Source: CAD feature listing. Evaluate the final solid. Frame: model axes, mm. A direction names the side the tool comes from. Coordinates: 2 decimals unless noted, no trailing zeros. Write each loop counter-clockwise with the first axis right and the second up, starting at its lowest first coordinate (ties: lowest second). Pieces come first, ordered by that corner, then holes. Notation, with made-up numbers: M -20,25 L 16,25 A13 cw 16,45 Z; hole C 39,-21 d9. An arc over 180 degrees is marked long. Write item = value, one per line. Start each with the question number.
1. Section query A-A (x = -20). Give the number of separate pieces and of enclosed holes in the cut face, then the cut area to 4 significant figures.
2. Section query C-C (z = 35). Output: boundary loops of the cut face in (x, y).
3. Access query for faces 4 (the face through (-5, 30, 53)), 5 (the face through (-33, 15, 37)), 6 (the face through (-8, 30, 42)), 7 (the face through (-20, 16, 47)), 8 (the face through (-33.5, 6, 51)). Directions: +Z, -Z, +X, -X, +Y, -Y. A direction counts if a zero-diameter tool reaches every point of the face in a straight line with its end or side. Return the directions, or none.
4. Pin query (flat end, axial travel): pin 1 Ø3.5 at (x, y) = (-8, 29.5) entering from +Z; pin 2 Ø2.5 at (x, y) = (-30, 7.5) entering from +Z; pin 3 Ø4 at (x, z) = (-16, 21.5) entering from +Y. Return the tip coordinate at first contact, or that it passes through.
5. Line query: line 1 along Z through (x, y) = (-9, 20); line 2 along Z through (x, y) = (-11.5, 31); line 3 along X through (y, z) = (3.5, 44.5). Output: solid intervals per line, ascending.
6. Pull-direction query (X, two-part tool) for faces 1 (the face through (0, 20, 28)), 2 (the face through (-30, 17, 31)), 3 (the face through (-9.748, 30.099, 55.028)); classes: pulls with the +X half, pulls with the -X half, needs draft (parallel to the pull), parting line crosses it, or undercut.
```python
from build123d import *

# Parameters (mm, degrees)
ESQUISSE1_W              = 40
ESQUISSE1_H              = 40
BOSS_EXTRU_1_DEPTH       = 50
ESQUISSE2_R              = 5
ENL_V_MAT_EXTRU_1_DEPTH  = 41
ESQUISSE3_R              = 5
ENL_V_MAT_EXTRU_2_DEPTH  = 41
ESQUISSE4_W              = 22
ESQUISSE4_H              = 14
ENL_V_MAT_EXTRU_3_DEPTH  = 29
ESQUISSE5_W              = 14
ESQUISSE5_H              = 20
ENL_V_MAT_EXTRU_4_DEPTH  = 29
ESQUISSE6_W              = 20
ESQUISSE6_H              = 14
ENL_V_MAT_EXTRU_5_DEPTH  = 24
ESQUISSE7_W              = 14
ESQUISSE7_H              = 22
ENL_V_MAT_EXTRU_6_DEPTH  = 24
ESQUISSE10_R             = 11
ENL_V_MAT_EXTRU_9_DEPTH  = 7
ESQUISSE11_R             = 12.5
ENL_V_MAT_EXTRU_10_DEPTH = 1.5
ESQUISSE14_R             = 11
ENL_V_MAT_EXTRU_11_DEPTH = 7
ESQUISSE15_R             = 12.5
ENL_V_MAT_EXTRU_12_DEPTH = 1.5
ESQUISSE16_W             = 40
ESQUISSE16_H             = 40
BOSS_EXTRU_2_DEPTH       = 7
ESQUISSE17_R             = 2.25
ENL_V_MAT_EXTRU_13_DEPTH = 15
ESQUISSE18_W             = 7
ESQUISSE18_H             = 3
ENL_V_MAT_EXTRU_14_DEPTH = 12
ESQUISSE19_W             = 3.5
ESQUISSE19_H             = 7.5
ENL_V_MAT_EXTRU_15_DEPTH = 12


with BuildPart() as part:
    # Esquisse1 → Boss.-Extru.1 (new body)
    with BuildSketch(Plane.XY):
        with Locations((-20, 20)):
            Rectangle(ESQUISSE1_W, ESQUISSE1_H)
    extrude(amount=BOSS_EXTRU_1_DEPTH)

    # Esquisse2 → Enlèv. mat.-Extru.1 (cut, through all)
    with BuildSketch(Plane(origin=(0, 40, 0), x_dir=(1, 0, 0), z_dir=(0, 1, 0))):
        with Locations(Location((-20, -15, 0), (0, 0, 270))):  # turned: the seam where the file's is
            Circle(ESQUISSE2_R)
    extrude(amount=-ENL_V_MAT_EXTRU_1_DEPTH, mode=Mode.SUBTRACT)

    # Esquisse3 → Enlèv. mat.-Extru.2 (cut, through all)
    with BuildSketch(Plane.ZY.offset(40)):
        with Locations((35, 20)):
            Circle(ESQUISSE3_R)
    extrude(amount=-ENL_V_MAT_EXTRU_2_DEPTH, mode=Mode.SUBTRACT)

    # Esquisse4 → Enlèv. mat.-Extru.3 (cut)
    with BuildSketch(Plane.ZY.offset(40)):
        with Locations((11, 20)):
            Rectangle(ESQUISSE4_W, ESQUISSE4_H)
    extrude(amount=-ENL_V_MAT_EXTRU_3_DEPTH, mode=Mode.SUBTRACT)

    # Esquisse5 → Enlèv. mat.-Extru.4 (cut)
    with BuildSketch(Plane.XZ):
        with Locations((-20, 35)):
            Rectangle(ESQUISSE5_W, ESQUISSE5_H)
    extrude(amount=-ENL_V_MAT_EXTRU_4_DEPTH, mode=Mode.SUBTRACT)

    # Esquisse6 → Enlèv. mat.-Extru.5 (cut)
    with BuildSketch(Plane(origin=(0, 0, 0), x_dir=(0, 0, -1), z_dir=(1, 0, 0))):
        with Locations((-15, 20)):
            Rectangle(ESQUISSE6_W, ESQUISSE6_H)
    extrude(amount=-ENL_V_MAT_EXTRU_5_DEPTH, mode=Mode.SUBTRACT)

    # Esquisse7 → Enlèv. mat.-Extru.6 (cut)
    with BuildSketch(Plane(origin=(0, 40, 0), x_dir=(1, 0, 0), z_dir=(0, 1, 0))):
        with Locations((-20, -39)):
            Rectangle(ESQUISSE7_W, ESQUISSE7_H)
    extrude(amount=-ENL_V_MAT_EXTRU_6_DEPTH, mode=Mode.SUBTRACT)

    # Esquisse10 → Enlèv. mat.-Extru.9 (cut)
    with BuildSketch(Plane(origin=(0, 40, 0), x_dir=(1, 0, 0), z_dir=(0, 1, 0))):
        with Locations(Location((-20, -15, 0), (0, 0, 270))):  # turned: the seam where the file's is
            Circle(ESQUISSE10_R)
    extrude(amount=-ENL_V_MAT_EXTRU_9_DEPTH, mode=Mode.SUBTRACT)

    # Esquisse11 → Enlèv. mat.-Extru.10 (cut)
    with BuildSketch(Plane(origin=(0, 40, 0), x_dir=(1, 0, 0), z_dir=(0, 1, 0))):
        with Locations(Location((-20, -15, 0), (0, 0, 270))):  # turned: the seam where the file's is
            Circle(ESQUISSE11_R)
    extrude(amount=-ENL_V_MAT_EXTRU_10_DEPTH, mode=Mode.SUBTRACT)

    # Esquisse14 → Enlèv. mat.-Extru.11 (cut)
    with BuildSketch(Plane.ZY.offset(40)):
        with Locations((35, 20)):
            Circle(ESQUISSE14_R)
    extrude(amount=-ENL_V_MAT_EXTRU_11_DEPTH, mode=Mode.SUBTRACT)

    # Esquisse15 → Enlèv. mat.-Extru.12 (cut)
    with BuildSketch(Plane.ZY.offset(40)):
        with Locations((35, 20)):
            Circle(ESQUISSE15_R)
    extrude(amount=-ENL_V_MAT_EXTRU_12_DEPTH, mode=Mode.SUBTRACT)

    # Esquisse16 → Boss.-Extru.2 (add)
    with BuildSketch(Plane.XY.offset(50)):
        with Locations((-20, 20)):
            Rectangle(ESQUISSE16_W, ESQUISSE16_H)
    extrude(amount=BOSS_EXTRU_2_DEPTH)

    # Esquisse17 → Enlèv. mat.-Extru.13 (cut)
    with BuildSketch(Plane.XY.offset(57)):
        with Locations((-30, 7.5)):
            Circle(ESQUISSE17_R)
        with Locations((-7.5, 30)):
            Circle(ESQUISSE17_R)
    extrude(amount=-ENL_V_MAT_EXTRU_13_DEPTH, mode=Mode.SUBTRACT)

    # Esquisse18 → Enlèv. mat.-Extru.14 (cut)
    with BuildSketch(Plane.XZ):
        with Locations((-30, 51.5)):
            Rectangle(ESQUISSE18_W, ESQUISSE18_H)
    extrude(amount=-ENL_V_MAT_EXTRU_14_DEPTH, mode=Mode.SUBTRACT)

    # Esquisse19 → Enlèv. mat.-Extru.15 (cut)
    with BuildSketch(Plane(origin=(0, 0, 0), x_dir=(0, 0, -1), z_dir=(1, 0, 0))):
        with Locations((-51.25, 30)):
            Rectangle(ESQUISSE19_W, ESQUISSE19_H)
    extrude(amount=-ENL_V_MAT_EXTRU_15_DEPTH, mode=Mode.SUBTRACT)


solid = part.part
```
Results are:
q1.separate_pieces = 5
q1.enclosed_holes = 0
q1.area = 694.5 mm^2
q2.outline = M -40,0 L -27,0 L -27,15 L -33,15 L -33,9 L -38.5,9 L -38.5,7.5 L -40,7.5 Z; M -40,32.5 L -38.5,32.5 L -38.5,31 L -33,31 L -33,25 L -27,25 L -27,40 L -40,40 Z; M -13,0 L 0,0 L 0,15 L -13,15 Z; M -13,25 L 0,25 L 0,40 L -13,40 Z
q3.face_4 = +X
q3.face_5 = -X
q3.face_6 = +Z
q3.face_7 = +Y
q3.face_8 = -Y
q4.pin_1 = 57
q4.pin_2 = 42
q4.pin_3 = 33
q5.line_1 = 0 to 5, 25 to 30, 40 to 57
q5.line_2 = 0 to 49.5, 53 to 57
q5.line_3 = -40 to -27, -13 to 0
q6.face_1 = pulls with the +X half
q6.face_2 = needs draft
q6.face_3 = undercut
